```python
from build123d import *

# Parameters (mm, degrees)
SKETCH1_R           = 3.3782
SKETCH1_R_2         = 1.905
SKETCH1_R_3         = 3.175
BOSS_EXTRUDE1_DEPTH = 6.35


with BuildPart() as part:
    # Sketch1 → Boss-Extrude1 (new body)
    with BuildSketch(Plane(origin=(0, 0, 0), x_dir=(1, 0, 0), z_dir=(0, 1, 0))):
        Polygon((25.4, 25.4), (25.4, 0), (127, 0), (127, 25.4), (152.4, 25.4), (152.4, 101.6), (127, 101.6), (127, 117.475), (25.4, 117.475), (25.4, 101.6), (0, 101.6), (0, 25.4), align=None)
        with Locations((12.7, 38.1)):
            Circle(SKETCH1_R, mode=Mode.SUBTRACT)
        with Locations((139.7, 38.1)):
            Circle(SKETCH1_R, mode=Mode.SUBTRACT)
        with Locations((12.7, 88.9)):
            Circle(SKETCH1_R, mode=Mode.SUBTRACT)
        with Locations((63.5, 92.075)):
            Circle(SKETCH1_R_2, mode=Mode.SUBTRACT)
        with Locations((63.5, 104.775)):
            Circle(SKETCH1_R_2, mode=Mode.SUBTRACT)
        with Locations((76.2, 66.675)):
            Circle(SKETCH1_R_3, mode=Mode.SUBTRACT)
        with Locations((88.9, 92.075)):
            Circle(SKETCH1_R_2, mode=Mode.SUBTRACT)
        with Locations((88.9, 104.775)):
            Circle(SKETCH1_R_2, mode=Mode.SUBTRACT)
        with Locations((139.7, 88.9)):
            Circle(SKETCH1_R, mode=Mode.SUBTRACT)
    extrude(amount=BOSS_EXTRUDE1_DEPTH)


solid = part.part
```
Verification items for the finished model (mm, model axes). A direction names the side the tool comes from. Coordinates: 2 decimals unless noted, no trailing zeros. Write each loop counter-clockwise with the first axis right and the second up, starting at its lowest first coordinate (ties: lowest second). Pieces come first, ordered by that corner, then holes. Notation, with made-up numbers: M 7,86.25 L 59,86.25 A12 cw 59,100.25 Z; hole C 5.5,67 d6. An arc over 180 degrees is marked long. One line per item, written item: value.
Item 1: Section check D-D, the plane z = -11. Record the boundary of the cut face in (x, y), plus the area to 3 significant figures.
Check sheet entries:
outline: M 25.4,0 L 127,0 L 127,6.35 L 25.4,6.35 Z
area: 645 mm^2
Item 2: Gauge pin test, flat ends, axial feed: pin 1 Ø3 at (y, z) = (2, -8) entering from +X; pin 2 Ø1.9 at (x, y) = (7.5, 4.5) entering from -Z; pin 3 Ø1.9 at (x, y) = (10, 3.5) entering from +Z. Record the tip position at first contact, or that the pin passes through.
Check sheet entries:
pin 1: stops at x = 127
pin 2: stops at z = -101.6
pin 3: stops at z = -25.4
Item 3: Scan lines: line 1 along Z through (x, y) = (88.9, 2) (3 decimals); line 2 along X through (y, z) = (3.75, -86.5); line 3 along Z through (x, y) = (11.5, 3.75). Record each from-to range of solid material in increasing order.
Check sheet entries:
line 1: z = -117.475 to -106.68, -102.87 to -93.98, -90.17 to 0
line 2: x = 0 to 10.32, 15.08 to 137.32, 142.08 to 152.4
line 3: z = -101.6 to -92.06, -85.74 to -41.26, -34.94 to -25.4
Item 4: Section check B-B, the plane z = -38.1. Record the boundary of the cut face in (x, y), plus the area to 3 significant figures.
Check sheet entries:
outline: M 0,0 L 9.32,0 L 9.32,6.35 L 0,6.35 Z; M 16.08,0 L 136.32,0 L 136.32,6.35 L 16.08,6.35 Z; M 143.08,0 L 152.4,0 L 152.4,6.35 L 143.08,6.35 Z
area: 882 mm^2
Item 5: Section check A-A, the plane x = 63.5. Record the boundary of the cut face in (y, z) (3 decimals), plus the area to 3 significant figures.
Check sheet entries:
outline: M 0,-117.475 L 6.35,-117.475 L 6.35,-106.68 L 0,-106.68 Z; M 0,-102.87 L 6.35,-102.87 L 6.35,-93.98 L 0,-93.98 Z; M 0,-90.17 L 6.35,-90.17 L 6.35,0 L 0,0 Z
area: 698 mm^2
Item 6: Access from +Z, -Z, +X, -X, +Y, -Y to the whole of each face (thin tool, end or side, straight path). Record for faces 4 (the flat face through (127, 3, -109)), 5 (the flat face through (75, 0, -60)), 6 (the flat face through (13, 3, -101.6)), 7 (the flat face through (127, 3, -13)).
Check sheet entries:
face 4: -Z, +X, +Y, -Y
face 5: +Z, -Z, +X, -X, -Y
face 6: -Z, -X, +Y, -Y
face 7: +Z, +X, +Y, -Y
Item 7: Mould release check, pull along X, two halves, no side actions. Record for faces 1 (the flat face through (152.4, 3, -63)), 2 (the cylindrical face through (87.4, 3.1, -90.9)), 3 (the flat face through (25.4, 3, -13)): pulls with the +X half, pulls with the -X half, needs draft (parallel to the pull), parting line crosses it, or undercut.
Check sheet entries:
face 1: pulls with the +X half
face 2: undercut
face 3: pulls with the -X half
Item 8: Section check C-C, the plane y = 4. State how many separate pieces and enclosed holes the cut face has, plus the area to 3 significant figures.
Check sheet entries:
separate pieces: 1
enclosed holes: 9
area: 15,600 mm^2
